CAD build for the part. Positions are in the model's coordinates, mm. Face numbers are marked on the shaded views. A direction names the side the tool comes from. Round coordinates to 2 decimals unless told otherwise and drop trailing zeros. Write each loop counter-clockwise with the first axis right and the second up, starting at its lowest first coordinate (ties: lowest second). Pieces come first, ordered by that corner, then holes. Notation, with made-up numbers: (49, -19) - (98, -19) arc R26 cw to (98, 2) - close; hole circle Ø1 at (1, -21). An arc over 180 degrees is marked (long way). Answer in a Markdown table with one row per item.
```python
from build123d import *
from build123d.topology import SkipClean

# Parameters (mm, degrees)
BOSS_EXTRUDE1_DEPTH      = 3.95
SHELL1_T                 = -1.2
SKETCH3_W                = 6.823927471
SKETCH3_H                = 5.581929969
CUT_EXTRUDE1_DEPTH       = 2.4
BOSS_EXTRUDE3_REACH      = 14.559
BOSS_EXTRUDE3_END_RADIUS = 43.712775366
BOSS_EXTRUDE3_START      = -1.8
SKETCH4_R                = 2.4
SKETCH4_R_2              = 1.9
CUT_EXTRUDE4_REACH       = 13.553
BOSS_EXTRUDE4_START      = -3.51
BOSS_EXTRUDE4_DEPTH      = 3.51
SHELL2_START             = 3.540892579
SHELL2_OUTLINE_W         = 7.9
SHELL2_OUTLINE_H         = 6.98035738
SHELL2_DEPTH             = 3.609652258
SHELL2_START_2           = 1.037208095
SHELL2_2_DEPTH           = 4.401988613
SHELL2_START_3           = -10.97
SHELL2_3_DEPTH           = 7.02
SHELL2_4_DEPTH           = 7.02
CUT_EXTRUDE5_DEPTH       = 22.359542769
SKETCH16_W               = 22.82
SKETCH16_H               = 1.2435468
CUT_EXTRUDE10_DEPTH      = 7.9
SKETCH17_W               = 3.486934667
SKETCH17_H               = 7.447231284
SKETCH17_W_2             = 3.517769968
CUT_EXTRUDE11_DEPTH      = 27.03272194
CUT_EXTRUDE12_DEPTH      = 18.123431779
CUT_EXTRUDE13_DEPTH      = 20.609163221
BOSS_EXTRUDE5_DEPTH      = 1.2
SKETCH23_W               = 3.213065333
SKETCH23_H               = 2.258477707
SKETCH23_W_2             = 3.182230032
BOSS_EXTRUDE6_DEPTH      = 1.2
BOSS_EXTRUDE7_START      = -1.2
BOSS_EXTRUDE7_DEPTH      = 1.2
CUT_EXTRUDE14_DEPTH      = 19.031936029


with BuildPart() as part:
    # Sketch1 → Boss-Extrude1 (new, symmetric)
    with BuildSketch(Plane.XY):
        with BuildLine():
            Line((7.9, 8.484439379), (7.9, 5.540892579))
            Line((7.9, 5.540892579), (7.9, 2.340892579))
            Line((7.9, 2.340892579), (0, 2.340892579))
            Line((0, 2.340892579), (0, 1.037208095))
            Line((0, 1.037208095), (-7.9, 1.037208095))
            Line((-7.9, 1.037208095), (-7.9, 4.036739959))
            ThreePointArc((-7.9, 4.036739959), (-0.204910293, 6.988512651), (7.9, 8.484439379))
        make_face()
    extrude(amount=BOSS_EXTRUDE1_DEPTH, both=True)

    # Shell1
    shell1_openings = [part.faces().sort_by_distance(p)[0] for p in [
        (-3.95, 1.037208095, 0),
    ]]
    offset(amount=SHELL1_T, openings=shell1_openings, kind=Kind.INTERSECTION)

    # Sketch3 → Cut-Extrude1 (cut)
    with BuildSketch(Plane.XZ.offset(-2.340892579)):
        with Locations((3.411963736, 0.021143674)):
            Rectangle(SKETCH3_W, SKETCH3_H)
    extrude(amount=-CUT_EXTRUDE1_DEPTH, mode=Mode.SUBTRACT)

    # Boss-Extrude3: up to this cylinder (the profile starts inside it)
    boss_extrude3_end = Plane(origin=(11.965039047, -36.243995073, 2.332118), z_dir=(0, 0, -1)) * Cylinder(BOSS_EXTRUDE3_END_RADIUS, 117.543550731, mode=Mode.PRIVATE)
    # Sketch4 → Boss-Extrude3 (add, up to the surface)
    with BuildSketch(Plane(origin=(0, 2.340892579, 0), x_dir=(-1, 0, 0), z_dir=(0, -1, 0)).offset(BOSS_EXTRUDE3_START), mode=Mode.PRIVATE) as boss_extrude3_sk1:
        with Locations(Location((-3.411963735, 0, 0), (0, 0, 90))):
            Circle(SKETCH4_R)
        with Locations(Location((-3.411963735, 0, 0), (0, 0, 90))):
            Circle(SKETCH4_R_2, mode=Mode.SUBTRACT)
    boss_extrude3_tool1 = extrude(boss_extrude3_sk1.sketch, amount=-BOSS_EXTRUDE3_REACH, mode=Mode.PRIVATE) & boss_extrude3_end
    add(boss_extrude3_tool1.solids().sort_by_distance((3.411964, 4.140893, 2.332118))[0])

    # Sketch7 → Cut-Extrude4 (cut, up to next)
    with BuildSketch(Plane(origin=(0, 1.037208095, 0), x_dir=(-1, 0, 0), z_dir=(0, -1, 0)), mode=Mode.PRIVATE) as cut_extrude4_sk1:
        Polygon((7.9, 3.95), (0, -3.95), (7.9, -3.95), align=None)
    cut_extrude4_tool1 = extrude(cut_extrude4_sk1.sketch, amount=-CUT_EXTRUDE4_REACH, mode=Mode.PRIVATE) & part.part
    add(cut_extrude4_tool1.solids().sort_by_distance((-5.266667, 1.037208, 1.316667))[0], mode=Mode.SUBTRACT)

    # Sketch8 → Boss-Extrude4 (add)
    with BuildSketch(Plane(origin=(0, 0, -7.46), x_dir=(-1, 0, 0), z_dir=(0, 0, -1)).offset(BOSS_EXTRUDE4_START)):
        with BuildLine():
            Line((-7.9, 7.189017048), (-7.9, 2.340892579))
            Line((-7.9, 2.340892579), (0, 2.340892579))
            Line((0, 2.340892579), (0, 1.037208095))
            Line((0, 1.037208095), (7.9, 1.037208095))
            Line((7.9, 1.037208095), (7.9, 4.036739959))
            ThreePointArc((7.9, 4.036739959), (0.204910293, 6.988512651), (-7.9, 8.484439379))
            Line((-7.9, 8.484439379), (-7.9, 7.189017048))
        make_face()
    extrude(amount=BOSS_EXTRUDE4_DEPTH)

    # Mirror1: part across plane


with BuildPart() as part_1:
    add(part.part)
    add(part.part.mirror(Plane(origin=(0, 0, -7.46), x_dir=(1, 0, 0), z_dir=(0, 0, -1))))

    # Shell2: read off the stored shape, not the designer's step
    # Shell2 outline → Shell2 (cut)
    with BuildSketch(Plane(origin=(0, 0, 0), x_dir=(1, 0, 0), z_dir=(0, 1, 0)).offset(SHELL2_START)):
        with Locations((2.75, 7.46)):
            Rectangle(SHELL2_OUTLINE_W, SHELL2_OUTLINE_H)
    extrude(amount=SHELL2_DEPTH, mode=Mode.SUBTRACT)

    # Shell2 2 outline → Shell2 2 (cut)
    with BuildSketch(Plane(origin=(0, 0, 0), x_dir=(1, 0, 0), z_dir=(0, 1, 0)).offset(SHELL2_START_2)):
        Polygon((-1.2, 3.95), (-1.2, 10.97), (-6.202943725, 10.97), (-6.7, 10.472943725), (-6.7, 4.447056275), (-6.202943725, 3.95), align=None)
    extrude(amount=SHELL2_2_DEPTH, mode=Mode.SUBTRACT)

    # Shell2 3 outline → Shell2 3 (cut)
    with BuildSketch(Plane.XY.offset(SHELL2_START_3)):
        with BuildLine():
            ThreePointArc((6.7, 7.150544837), (3.582625992, 6.65754198), (0.508949666, 5.940892579))
            Line((0.508949666, 5.940892579), (6.7, 5.940892579))
            Line((6.7, 5.940892579), (6.7, 7.150544837))
        make_face()
    extrude(amount=SHELL2_3_DEPTH, mode=Mode.SUBTRACT)

    # Shell2 4 outline → Shell2 4 (add)
    with SkipClean():  # the faces are left unmerged after this step: merging them gives an invalid solid
        with BuildSketch(Plane.XY.offset(SHELL2_START_3)):
            with BuildLine():
                ThreePointArc((-4.75826547, 5.439196708), (-5.7340289, 5.034333198), (-6.7, 4.606631708))
                Line((-6.7, 4.606631708), (-6.7, 3.283502287))
                ThreePointArc((-6.7, 3.283502287), (-3.986456885, 4.454364939), (-1.2, 5.439196708))
                Line((-1.2, 5.439196708), (-4.75826547, 5.439196708))
            make_face()
            with BuildLine():
                ThreePointArc((0.386122992, 7.150544837), (-0.40902625, 6.930533287), (-1.2, 6.69595297))
                Line((-1.2, 6.69595297), (-1.2, 5.439196708))
                ThreePointArc((-1.2, 5.439196708), (2.710357921, 6.477868269), (6.7, 7.150544837))
                Line((6.7, 7.150544837), (0.386122992, 7.150544837))
            make_face()
        extrude(amount=SHELL2_4_DEPTH)
    add(part_1.part.scale(1), mode=Mode.REPLACE)  # the faces are merged on a copy

    # Sketch10 → Cut-Extrude5 (cut, through all)
    with BuildSketch(Plane(origin=(0, 2.340892579, 0), x_dir=(-1, 0, 0), z_dir=(0, -1, 0))):
        Polygon((1.2, 12.17), (1.2, 10.97), (6.202943725, 10.97), (6.7, 10.472943725), (7.9, 10.97), (6.7, 12.17), align=None)
        Polygon((1.2, 2.75), (6.7, 2.75), (7.9, 3.95), (6.7, 4.447056275), (6.202943725, 3.95), (1.2, 3.95), align=None)
    extrude(amount=CUT_EXTRUDE5_DEPTH, mode=Mode.SUBTRACT)

    # Sketch16 → Cut-Extrude10 (cut)
    with BuildSketch(Plane(origin=(7.9, 0, 0), x_dir=(0, 0, -1), z_dir=(1, 0, 0))):
        with Locations((7.46, 2.962665979)):
            Rectangle(SKETCH16_W, SKETCH16_H)
    extrude(amount=-CUT_EXTRUDE10_DEPTH, mode=Mode.SUBTRACT)

    # Sketch17 → Cut-Extrude11 (cut, through all)
    with BuildSketch(Plane(origin=(7.9, 0, 0), x_dir=(0, 0, -1), z_dir=(1.0, -1.5823538232397524e-12, 0))):
        with Locations((-2.206532667, 4.760823737)):
            Rectangle(SKETCH17_W, SKETCH17_H)
        with Locations((17.111115016, 4.760823737)):
            Rectangle(SKETCH17_W_2, SKETCH17_H)
    extrude(amount=-CUT_EXTRUDE11_DEPTH, mode=Mode.SUBTRACT)

    # Sketch18 → Cut-Extrude12 (cut, through all)
    with BuildSketch(Plane.XY.offset(-2.75)):
        with BuildLine():
            Line((-1.2, 2.340892579), (-6.7, 2.340892579))
            Line((-6.7, 2.340892579), (-6.7, 3.283502287))
            ThreePointArc((-6.7, 3.283502287), (-3.986456885, 4.454364939), (-1.2, 5.439196708))
            Line((-1.2, 5.439196708), (-1.2, 3.540892579))
            Line((-1.2, 3.540892579), (-1.2, 2.340892579))
        make_face()
    extrude(amount=-CUT_EXTRUDE12_DEPTH, mode=Mode.SUBTRACT)

    # Sketch19 → Cut-Extrude13 (cut, through all)
    with BuildSketch(Plane.XY.offset(0.463065333)):
        with BuildLine():
            Line((0, 5.799370286), (0, 3.540892579))
            Line((0, 3.540892579), (6.823927471, 3.584439379))
            Line((6.823927471, 3.584439379), (6.823927471, 7.181547539))
            ThreePointArc((6.823927471, 7.181547539), (3.39019483, 6.597933861), (0, 5.799370286))
        make_face()
    extrude(amount=-CUT_EXTRUDE13_DEPTH, mode=Mode.SUBTRACT)

    # Sketch20 → Boss-Extrude5 (add)
    with BuildSketch(Plane(origin=(0, 0, 0), x_dir=(0, 0, -1), z_dir=(1, 0, 0))):
        Polygon((3.96982131, 3.540892579), (3.953429775, 6.436658409), (10.966345521, 6.396961672), (10.95017869, 3.540892579), align=None)
    extrude(amount=-BOSS_EXTRUDE5_DEPTH)

    # Sketch23 → Boss-Extrude6 (add)
    with BuildSketch(Plane(origin=(0, 0, 0), x_dir=(0, 0, -1), z_dir=(1, 0, 0))):
        with Locations((1.143467334, 4.670131432)):
            Rectangle(SKETCH23_W, SKETCH23_H)
        with Locations((13.761115016, 4.670131432)):
            Rectangle(SKETCH23_W_2, SKETCH23_H)
    extrude(amount=-BOSS_EXTRUDE6_DEPTH)

    # Sketch25 → Boss-Extrude7 (add)
    with BuildSketch(Plane.XY.offset(0.463065333).offset(BOSS_EXTRUDE7_START)):
        with BuildLine():
            Line((6.823927471, 3.584439379), (6.823927471, 7.181547539))
            ThreePointArc((6.823927471, 7.181547539), (3.384337724, 6.626850897), (0, 5.799370286))
            Line((0, 5.799370286), (0, 3.584439379))
            Line((0, 3.584439379), (6.823927471, 3.584439379))
        make_face()
        with BuildLine():
            Line((-6.7, 3.283502287), (-1.2, 3.283502287))
            Line((-1.2, 3.283502287), (-1.2, 5.439196708))
            ThreePointArc((-1.2, 5.439196708), (-3.986456885, 4.454364939), (-6.7, 3.283502287))
        make_face()
    boss_extrude7 = extrude(amount=BOSS_EXTRUDE7_DEPTH)

    # Sketch28 → Cut-Extrude14 (cut, through all)
    with BuildSketch(Plane.XZ.offset(-3.283502287)):
        Polygon((-4.686934667, -0.736934667), (-3.437061956, 0.463065333), (-6.7, 0.463065333), (-6.7, -0.736934667), align=None)
    cut_extrude14 = extrude(amount=-CUT_EXTRUDE14_DEPTH, mode=Mode.SUBTRACT)

    # Mirror2: Boss-Extrude7, Cut-Extrude14 across plane
    add(boss_extrude7.mirror(Plane(origin=(0, 0, -7.46), x_dir=(1, 0, 0), z_dir=(0, 0, -1))))
    add(cut_extrude14.mirror(Plane(origin=(0, 0, -7.46), x_dir=(1, 0, 0), z_dir=(0, 0, -1))), mode=Mode.SUBTRACT)


solid = part_1.part
```
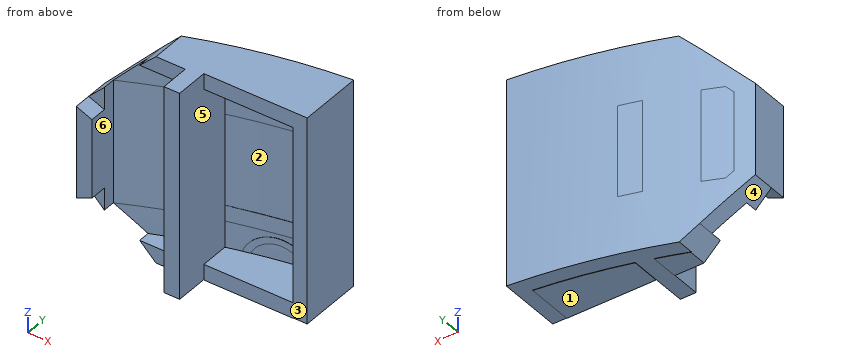
Q1. Drill centre lines: line 1 (Z direction, x = 2.75, y = 4.5); line 2 (X direction, y = 2.75, z = -7.75); line 3 (Z direction, x = -1.5, y = 6.25). Where is each one in solid material? Low to high.
Computed:
| item | result |
|---|---|
| line 1 | z = -15.38 to -14.18, -0.74 to 0.46 |
| line 2 | x = -7.9 to -6.7, -1.2 to 0 |
| line 3 | z = -15.35 to 0.46 |
Q2. Pull direction Z, two halves, no side cores. Call the marked faces 4, 5 and 6: released by +Z, released by -Z, zero draft, split by the parting line, or undercut.
Computed:
| item | result |
|---|---|
| face 4 | released by -Z |
| face 5 | undercut |
| face 6 | zero draft |
Q3. Flat gauge pins, fed straight in: pin 1 (1.8 mm diameter, centred on y = 5.5, z = -4.5, fed in from -X); pin 2 (8 mm diameter, centred on x = 1.5, z = -13.5, fed in from +Y); pin 3 (1.8 mm diameter, centred on y = 2, z = -8.5, fed in from +X). Where does each tip first touch, or does it go through?
Computed:
| item | result |
|---|---|
| pin 1 | stops at x = -6.71 |
| pin 2 | stops at y = 8.2 |
| pin 3 | stops at x = 0 |
Q4. Saw through at D-D on y = 5.25. Count the separate pieces of the cut face and the enclosed holes in it, then the cut area to 3 significant figures.
Computed:
| item | result |
|---|---|
| separate pieces | 1 |
| enclosed holes | 2 |
| area | 105 mm2 |
Q5. Saw through at A-A on z = -7.5. List the corners of the cut face in (x, y), then the cut area to 3 significant figures.
Computed:
| item | result |
|---|---|
| outline | (-7.9, 1.04) - (-6.7, 1.04) - (-6.7, 3.28) arc R43.71 cw to (-1.2, 5.44) - (-1.2, 1.04) - (0, 1.04) - (0, 5.8) arc R43.71 cw to (5.88, 7.04) arc R55.31 cw to (6.82, 7.18) - (6.82, 3.58) - (7.9, 3.58) - (7.9, 8.48) arc R44.91 ccw to (0.39, 7.15) arc R44.91 ccw to (-1.2, 6.7) arc R44.91 ccw to (-7.9, 4.04) - close |
| area | 31.6 mm2 |
Q6. 3-axis set-ups, long thin cutter, end or side, ignore diameter. For the marked faces 1, 2 and 3: which of +Z, -Z, +X, -X, +Y, -Y reach the whole face in a straight line?
Computed:
| item | result |
|---|---|
| face 1 | -Z, +X, -X, +Y, -Y |
| face 2 | -Y |
| face 3 | +Z, -Z, +X, -Y |
